from build123d import *

# Parameters (mm, degrees)
BOSS_EXTRUDE1_DEPTH = 165
SKETCH3_W           = 30
SKETCH3_H           = 32
BOSS_EXTRUDE2_DEPTH = 2
SKETCH4_W           = 30
SKETCH4_H           = 32
BOSS_EXTRUDE3_DEPTH = 2
BOSS_EXTRUDE4_START = 10
BOSS_EXTRUDE4_DEPTH = 10
CUT_EXTRUDE1_DEPTH  = 10
BOSS_EXTRUDE6_DEPTH = 15
CUT_EXTRUDE2_DEPTH  = 15
BOSS_EXTRUDE7_DEPTH = 121
CUT_EXTRUDE3_DEPTH  = 121
SKETCH13_W          = 169
SKETCH13_H          = 30
CUT_EXTRUDE5_DEPTH  = 3
SKETCH14_W          = 169
SKETCH14_H          = 30
BOSS_EXTRUDE8_DEPTH = 3
SKETCH12_W          = 28
SKETCH12_H          = 2
CUT_EXTRUDE6_DEPTH  = 168
SKETCH16_W          = 165
SKETCH16_H          = 26
CUT_EXTRUDE7_DEPTH  = 3
CUT_EXTRUDE8_DEPTH  = 1.5
CUT_EXTRUDE9_DEPTH  = 3
SKETCH20_W          = 169
SKETCH20_H          = 30
BOSS_EXTRUDE9_DEPTH = 1
SKETCH21_W          = 165
SKETCH21_H          = 26
CUT_EXTRUDE10_DEPTH = 1
FILLET1_START       = -16
FILLET1_DEPTH       = 35
FILLET1_2_DEPTH     = 32
FILLET2_R           = 1
CUT_EXTRUDE11_DEPTH = 12


with BuildPart() as part:
    # Sketch2 → Boss-Extrude1 (new body)
    with BuildSketch(Plane(origin=(0, 0, 0), x_dir=(0, 0, -1), z_dir=(1, 0, 0))):
        with BuildLine():
            Line((-13, 0), (-13, 17))
            Line((-13, 17), (-15, 17))
            Line((-15, 17), (-15, -15))
            Line((-15, -15), (15, -15))
            Line((15, -15), (15, 17))
            Line((15, 17), (13, 17))
            Line((13, 17), (13, 0))
            ThreePointArc((13, 0), (0, -13), (-13, 0))
        make_face()
    extrude(amount=BOSS_EXTRUDE1_DEPTH)

    # Sketch3 → Boss-Extrude2 (add)
    with BuildSketch(Plane(origin=(165, 0, 0), x_dir=(0, 0, -1), z_dir=(1, 0, 0))):
        with Locations((0, 1)):
            Rectangle(SKETCH3_W, SKETCH3_H)
    extrude(amount=BOSS_EXTRUDE2_DEPTH)

    # Sketch4 → Boss-Extrude3 (add)
    with BuildSketch(Plane.ZY):
        with Locations((0, 1)):
            Rectangle(SKETCH4_W, SKETCH4_H)
    extrude(amount=BOSS_EXTRUDE3_DEPTH)

    # Sketch5 → Boss-Extrude4 (add)
    with BuildSketch(Plane.ZY.offset(-165).offset(BOSS_EXTRUDE4_START)):
        with BuildLine():
            Line((-13, 17), (-13, 0))
            ThreePointArc((-13, 0), (0, -13), (13, 0))
            Line((13, 0), (13, 17))
            Line((13, 17), (-13, 17))
        make_face()
    extrude(amount=-BOSS_EXTRUDE4_DEPTH)

    # Sketch6 → Cut-Extrude1 (cut)
    with BuildSketch(Plane.ZY.offset(-155)):
        with BuildLine():
            Line((-2, 0), (-2, 17))
            Line((-2, 17), (2, 17))
            Line((2, 17), (2, 0))
            ThreePointArc((2, 0), (0, -2), (-2, 0))
        make_face()
    extrude(amount=-CUT_EXTRUDE1_DEPTH, mode=Mode.SUBTRACT)

    # Sketch8 → Boss-Extrude6 (add)
    with BuildSketch(Plane(origin=(0, 0, 0), x_dir=(0, 0, -1), z_dir=(1, 0, 0))):
        with BuildLine():
            Line((13, 0), (13, 17))
            Line((13, 17), (-13, 17))
            Line((-13, 17), (-13, 0))
            ThreePointArc((-13, 0), (0, -13), (13, 0))
        make_face()
    extrude(amount=BOSS_EXTRUDE6_DEPTH)

    # Sketch9 → Cut-Extrude2 (cut)
    with BuildSketch(Plane(origin=(15, 0, 0), x_dir=(0, 0, -1), z_dir=(1, 0, 0))):
        with BuildLine():
            Line((-2.125, 0), (-2.125, 17))
            Line((-2.125, 17), (2.125, 17))
            Line((2.125, 17), (2.125, 0))
            ThreePointArc((2.125, 0), (0, -2.125), (-2.125, 0))
        make_face()
    extrude(amount=-CUT_EXTRUDE2_DEPTH, mode=Mode.SUBTRACT)

    # Sketch10 → Boss-Extrude7 (add)
    with BuildSketch(Plane(origin=(15, 0, 0), x_dir=(0, 0, -1), z_dir=(1, 0, 0))):
        with BuildLine():
            Line((13, 0), (13, 17))
            Line((13, 17), (-13, 17))
            Line((-13, 17), (-13, 0))
            ThreePointArc((-13, 0), (0, -13), (13, 0))
        make_face()
    extrude(amount=BOSS_EXTRUDE7_DEPTH)

    # Sketch11 → Cut-Extrude3 (cut)
    with BuildSketch(Plane(origin=(136, 0, 0), x_dir=(0, 0, -1), z_dir=(1, 0, 0))):
        with BuildLine():
            Line((-8.5, 0), (-8.5, 17))
            Line((-8.5, 17), (8.5, 17))
            Line((8.5, 17), (8.5, 0))
            ThreePointArc((8.5, 0), (0, -8.5), (-8.5, 0))
        make_face()
    extrude(amount=-CUT_EXTRUDE3_DEPTH, mode=Mode.SUBTRACT)

    # Sketch13 → Cut-Extrude5 (cut)
    with BuildSketch(Plane(origin=(0, 17, 0), x_dir=(1, 0, 0), z_dir=(0, 1, 0))):
        with Locations((82.5, 0)):
            Rectangle(SKETCH13_W, SKETCH13_H)
    extrude(amount=-CUT_EXTRUDE5_DEPTH, mode=Mode.SUBTRACT)

    # Sketch14 → Boss-Extrude8 (add)
    with BuildSketch(Plane(origin=(0, 14, 0), x_dir=(1, 0, 0), z_dir=(0, 1, 0))):
        with Locations((82.5, 0)):
            Rectangle(SKETCH14_W, SKETCH14_H)
    extrude(amount=BOSS_EXTRUDE8_DEPTH)

    # Sketch12 → Cut-Extrude6 (cut)
    with BuildSketch(Plane(origin=(167, 0, 0), x_dir=(0, 0, -1), z_dir=(1, 0, 0))):
        with Locations((0, 15)):
            Rectangle(SKETCH12_W, SKETCH12_H)
    extrude(amount=-CUT_EXTRUDE6_DEPTH, mode=Mode.SUBTRACT)

    # Sketch16 → Cut-Extrude7 (cut)
    with BuildSketch(Plane(origin=(0, 17, 0), x_dir=(1, 0, 0), z_dir=(0, 1, 0))):
        with Locations((82.5, 0)):
            Rectangle(SKETCH16_W, SKETCH16_H)
    extrude(amount=-CUT_EXTRUDE7_DEPTH, mode=Mode.SUBTRACT)

    # Sketch17 → Cut-Extrude8 (cut)
    with BuildSketch(Plane(origin=(136, 0, 0), x_dir=(0, 0, -1), z_dir=(1, 0, 0))):
        with BuildLine():
            Line((13, 14), (13, 0))
            ThreePointArc((13, 0), (0, -13), (-13, 0))
            Line((-13, 0), (-13, 14))
            Line((-13, 14), (-8.5, 14))
            Line((-8.5, 14), (-8.5, 0))
            ThreePointArc((-8.5, 0), (0, -8.5), (8.5, 0))
            Line((8.5, 0), (8.5, 14))
            Line((8.5, 14), (13, 14))
        make_face()
    extrude(amount=-CUT_EXTRUDE8_DEPTH, mode=Mode.SUBTRACT)

    # Sketch18 → Cut-Extrude9 (cut)
    with BuildSketch(Plane(origin=(15, 0, 0), x_dir=(0, 0, -1), z_dir=(1, 0, 0))):
        with BuildLine():
            Line((8.5, 0), (8.5, 14))
            Line((8.5, 14), (2.125, 14))
            Line((2.125, 14), (2.125, 0))
            ThreePointArc((2.125, 0), (0, -2.125), (-2.125, 0))
            Line((-2.125, 0), (-2.125, 14))
            Line((-2.125, 14), (-8.5, 14))
            Line((-8.5, 14), (-8.5, 0))
            ThreePointArc((-8.5, 0), (0, -8.5), (8.5, 0))
        make_face()
    extrude(amount=-CUT_EXTRUDE9_DEPTH, mode=Mode.SUBTRACT)

    # Sketch20 → Boss-Extrude9 (add)
    with BuildSketch(Plane(origin=(0, 17, 0), x_dir=(1, 0, 0), z_dir=(0, 1, 0))):
        with Locations((82.5, 0)):
            Rectangle(SKETCH20_W, SKETCH20_H)
    extrude(amount=BOSS_EXTRUDE9_DEPTH)

    # Sketch21 → Cut-Extrude10 (cut)
    with BuildSketch(Plane(origin=(0, 18, 0), x_dir=(1, 0, 0), z_dir=(0, 1, 0))):
        with Locations((82.5, 0)):
            Rectangle(SKETCH21_W, SKETCH21_H)
    extrude(amount=-CUT_EXTRUDE10_DEPTH, mode=Mode.SUBTRACT)

    # Fillet1: read off the stored shape, not the designer's step
    # Fillet1 outline → Fillet1 (cut)
    with BuildSketch(Plane(origin=(0, 0, 0), x_dir=(1, 0, 0), z_dir=(0, 1, 0)).offset(FILLET1_START)):
        with BuildLine():
            Line((-2, 15), (-2, 14))
            ThreePointArc((-2, 14), (-1.707106781, 14.707106781), (-1, 15))
            Line((-1, 15), (-2, 15))
        make_face()
        with BuildLine():
            ThreePointArc((-1, -15), (-1.707106781, -14.707106781), (-2, -14))
            Line((-2, -14), (-2, -15))
            Line((-2, -15), (-1, -15))
        make_face()
        with BuildLine():
            Line((167, 15), (166, 15))
            ThreePointArc((166, 15), (166.707106781, 14.707106781), (167, 14))
            Line((167, 14), (167, 15))
        make_face()
        with BuildLine():
            ThreePointArc((167, -14), (166.707106781, -14.707106781), (166, -15))
            Line((166, -15), (167, -15))
            Line((167, -15), (167, -14))
        make_face()
    extrude(amount=FILLET1_DEPTH, mode=Mode.SUBTRACT)

    # Fillet1 2 outline → Fillet1 2 (cut)
    with BuildSketch(Plane.XY.offset(FILLET1_START)):
        with BuildLine():
            Line((167, 18), (166, 18))
            ThreePointArc((166, 18), (166.707106781, 17.707106781), (167, 17))
            Line((167, 17), (167, 18))
        make_face()
        with BuildLine():
            ThreePointArc((-2, 17), (-1.707106781, 17.707106781), (-1, 18))
            Line((-1, 18), (-2, 18))
            Line((-2, 18), (-2, 17))
        make_face()
    extrude(amount=FILLET1_2_DEPTH, mode=Mode.SUBTRACT)

    # Fillet2
    fillet2_edges = [part.edges().sort_by_distance(p)[0] for p in [
        (0, 17, 13),
        (0, 17, -13),
        (165, 17, -13),
        (165, 17, 13),
    ]]
    fillet(fillet2_edges, radius=FILLET2_R)

    # Sketch22 → Cut-Extrude11 (cut)
    with BuildSketch(Plane(origin=(12, 0, 0), x_dir=(0, 0, -1), z_dir=(1, 0, 0))):
        with BuildLine():
            Line((-2.125, 0), (-2.125, -8.230089611))
            ThreePointArc((-2.125, -8.230089611), (0, -8.5), (2.125, -8.230089611))
            Line((2.125, -8.230089611), (2.125, 0))
            ThreePointArc((2.125, 0), (0, -2.125), (-2.125, 0))
        make_face()
    extrude(amount=-CUT_EXTRUDE11_DEPTH, mode=Mode.SUBTRACT)


solid = part.part
Verification items for the finished model (mm, model axes). A direction names the side the tool comes from. Give positions to 0.01 mm unless a question says otherwise; leave off trailing zeros. Loops run counter-clockwise (first coordinate to the right, second up) from the corner with the lowest first, then second, coordinate; pieces in that order, holes last.
1. Cross-section at A-A on z = 0. Record the cut outline in (x, y).
Derived:
outline: (-2, -15) - (167, -15) - (167, 14) - (165, 14) - (165, -2) - (155, -2) - (155, -13) - (134.5, -13) - (134.5, -8.5) - (0, -8.5) - (0, 14) - (-1, 14) - (-1, 16) - (0, 16) - (0, 18) - (-1, 18) arc R1 ccw to (-2, 17) - close; (165, 16) - (167, 16) - (167, 17) arc R1 ccw to (166, 18) - (165, 18) - close
2. Cross-section at C-C on x = 83. Record the cut outline in (y, z), and give its area (3 significant figures).
Derived:
outline: (-15, -15) - (18, -15) - (18, -13) - (16, -13) - (16, -14) - (14, -14) - (14, -8.5) - (0, -8.5) arc R8.5 cw to (0, 8.5) - (14, 8.5) - (14, 14) - (16, 14) - (16, 13) - (18, 13) - (18, 15) - (-15, 15) - close
area: 531 mm2
3. Go/stop test with flat-tipped pins: P1, Ø1, axis at x = 29, z = -11, coming from the +Y side; P2, Ø6, axis at x = 109.5, z = 1, coming from the +Y side; P3, Ø4, axis at x = 108.5, z = 3.5, coming from the +Y side. Record where each tip stops, or that it passes through.
Derived:
P1: stops at y = 14
P2: stops at y = -7.5
P3: stops at y = -6.48
4. Release check for a two-part mould opening along Z. For faces 3 (the flat face through (167, -1, 0)), 4 (the flat face through (81, 1, 15)), 5 (the flat face through (160, 7, 2)) record: +Z half, -Z half, draft (parallel to the pull), parting line (faces both ways), or undercut.
Derived:
face 3: draft
face 4: +Z half
face 5: undercut
5. Cross-section at B-B on y = 7.5. Record the cut outline in (x, z) (3 decimals), and give its area (3 significant figures).
Derived:
outline: (-2, -14) arc R1 ccw to (-1, -15) - (166, -15) arc R1 ccw to (167, -14) - (167, 14) arc R1 ccw to (166, 15) - (-1, 15) arc R1 ccw to (-2, 14) - close; hole (0, -2.125) - (12, -2.125) - (12, -8.5) - (134.5, -8.5) - (134.5, -13) - (155, -13) - (155, -2) - (165, -2) - (165, 2) - (155, 2) - (155, 13) - (134.5, 13) - (134.5, 8.5) - (12, 8.5) - (12, 2.125) - (0, 2.125) - close
area: 2,360 mm2
6. Tool access check on faces 1 (the cylindrical face through (160, -2, 0)), 2 (the flat face through (81, 1, -15)). Record the directions out of +Z, -Z, +X, -X, +Y, -Y that give a thin tool (end or side, any length) a straight path to the whole face; none if there is none.
Derived:
face 1: +Y
face 2: -Z, +X, -X, +Y, -Y
7. Cross-section at D-D on z = -10.5. Record the cut outline in (x, y).
Derived:
outline: (-2, -15) - (167, -15) - (167, 14) - (155, 14) - (155, -7.66) - (134.5, -7.66) - (134.5, 14) - (-1, 14) - (-1, 16) - (0, 16) - (0, 18) - (-1, 18) arc R1 ccw to (-2, 17) - close; (165, 16) - (167, 16) - (167, 17) arc R1 ccw to (166, 18) - (165, 18) - close
8. Material ranges on probe 1 along Z at (x, y) = (41, 16.5); probe 2 along Z at (x, y) = (28, 0.5); probe 3 along X at (y, z) = (3.5, -7.5), recorded low to high.
Derived:
probe 1: z = -15 to -13, 13 to 15
probe 2: z = -15 to -8.5, 8.5 to 15
probe 3: x = -2 to 12, 155 to 167
